Autodesk Inventor part; units mm, degrees
ref_plane "YZ Plane" through (0, 0, 0) normal (1, 0, 0) x (0, 1, 0)
ref_plane "XZ Plane" through (0, 0, 0) normal (0, 1, 0) x (-1, 0, 0)
ref_plane "XY Plane" through (0, 0, 0) normal (0, 0, 1) x (1, 0, 0)
sketch "Sketch1" plane through (0, 0, 0) normal (0, 0, 1) x (1, 0, 0)
  line L0 (-77.055, 89.1324) -> (76.1519, 89.1324)
  line L1 (139.6519, 27.5351) -> (139.6519, -25.4)
  line L2 (76.2, -88.852) -> (-88.4125, -88.852)
  line L3 (-139.7639, 88.9233) -> (139.6519, -88.852) construction
  line L4 (139.6519, 89.1324) -> (-139.2125, -88.852) construction
  line L5 (139.6519, 0.1402) -> (139.6519, 27.5351)
  line L6 (139.6519, 0.1402) -> (139.6519, -25.4)
  line L7 (139.6519, 0.1402) -> (139.6519, -25.4)
  line L8 (139.6519, -25.4) -> (76.2, -88.852)
  line L9 (139.6519, 27.5351) -> (76.1519, 89.1324)
  arc A0 (-139.0653, -41.9162) -> (-88.4125, -88.852) centre (-88.4125, -38.052) ccw
  line L10 (-137.5184, -35.1177) -> (-101.1125, 27.9391)
  line L11 (-139.2125, -38.052) -> (-66.4007, -38.052) construction
  line L12 (-101.1125, 27.9391) -> (-101.1125, 65.0749)
  arc A1 (-137.5184, -35.1177) -> (-139.0653, -41.9162) centre (-127.298, -41.0185) ccw
  line L13 (-77.055, 89.1324) -> (-101.1125, 65.0749)
  line L14 (-77.055, 89.1324) -> (-42.3901, 89.1324) construction
  point P0 (0, 0)
  dimension "d9" = 50.8
extrude "Extrusion1" add sketch "Sketch1" along normal mid plane 203.2
sketch "Sketch2" plane through (-77.055, 89.1324, 101.6) normal (0, 1, 0) x (1, 0, 0)
  circle A0 centre (77.055, 101.6) radius 25.4
  dimension "d16" = 50.8
extrude "Extrusion2" cut sketch "Sketch2" against normal blind 38.1
sketch "Sketch4" plane through (0, 0, 101.6) normal (0, 0, 1) x (1, 0, 0)
  circle A0 centre (0, 0) radius 19.05
  dimension "d22" = 38.1
sketch "Sketch5" plane through (0, 0, -101.6) normal (0, 0, -1) x (-1, 0, 0)
  circle A0 centre (0, 0) radius 19.05
  dimension "d23" = 38.1
extrude "Extrusion4" add sketch "Sketch5" along normal blind 203.2
extrude "Extrusion5" add sketch "Sketch4" along normal blind 203.2
sketch "Sketch6" plane through (-101.1125, 27.9391, 101.6) normal (-1, 0, 0) x (0, 0, 1)
  line L0 (-127, 12.4705) -> (-75.6804, 12.4705)
  line L1 (-127, 12.4705) -> (-76.2, 12.4705)
  line L2 (-76.2, 12.4705) -> (-76.2, -116.9301)
  line L3 (-76.2, -116.9301) -> (-127, -116.9301)
  line L4 (-127, -116.9301) -> (-127, 12.4705)
  point P0 (-101.6, -27.9391)
extrude "Extrusion6" cut sketch "Sketch6" along normal blind 38.1 and the other way blind 19.05
sketch "Sketch7" plane through (-101.1125, 27.9391, -25.4) normal (0, 0, 1) x (1, 0, 0)
  circle A0 centre (-3.8712, -78.6483) radius 12.7
  point P0 (101.1125, -27.9391)
  dimension "d34" = 25.4
extrude "Extrusion7" add sketch "Sketch7" along normal blind 50.8
sketch "Sketch8" plane through (-101.1125, 27.9391, -25.4) normal (0, 0, 1) x (1, 0, 0)
  line L0 (19.05, -116.7911) -> (19.05, 12.4705)
  arc A0 (19.05, -116.7911) -> (19.05, 12.4705) centre (-100.0567, -52.1603) ccw
  point P0 (101.1125, -27.9391)
extrude "Extrusion8" cut sketch "Sketch8" along normal blind 50.8
sketch "Sketch10" plane through (0, 51.0324, 0) normal (0, 1, 0) x (1, 0, 0)
  circle A0 centre (0, 0) radius 25.4
  circle A1 centre (0, 0) radius 31.75
  dimension "d42" = 63.5
extrude "Extrusion10" cut sketch "Sketch10" along normal blind 5.08
properties part number "center piece"
Geometry check sheet. Reference: the model listing, model coordinates, mm. A direction names the side the tool comes from. Give positions to 0.01 mm unless a question says otherwise; leave off trailing zeros. Order: outer loops, then holes, each group sorted by start corner. A loop starts at its lowest first (then second) coordinate and runs counter-clockwise, first axis right, second up.
1. Sectioned sample at B-B (y = 0). Record the boundary of the cut face in (x, z), then the cut area to 3 significant figures.
Completed:
outline: (-117.24, -101.6) - (-19.05, -101.6) - (-19.05, -304.8) - (19.05, -304.8) - (19.05, -101.6) - (139.65, -101.6) - (139.65, 101.6) - (19.05, 101.6) - (19.05, 304.8) - (-19.05, 304.8) - (-19.05, 101.6) - (-117.24, 101.6) - (-117.24, 25.4) - (-67.84, 25.4) - (-67.84, -25.4) - (-117.24, -25.4) - close
area: 65,200 mm2
2. Draft check along X on faces 3 (the face through (-88.92, 77.27, -1.42)), 4 (the face through (0, 51.032, 0)), 5 (the face through (-6.883, 53.537, -30.995)), 6 (the face through (108.37, -56.68, -1.42)). Enter one of: pulls with the +X half, pulls with the -X half, needs draft (parallel to the pull), parting line crosses it, or undercut.
Completed:
face 3: pulls with the -X half
face 4: undercut
face 5: undercut
face 6: pulls with the +X half
3. Sectioned sample at A-A (x = 0). Record the boundary of the cut face in (y, z), then the cut area to 3 significant figures.
Completed:
outline: (-88.85, -101.6) - (-19.05, -101.6) - (-19.05, -304.8) - (19.05, -304.8) - (19.05, -101.6) - (89.13, -101.6) - (89.13, -25.4) - (56.11, -25.4) - (56.11, -31.75) - (51.03, -31.75) - (51.03, 31.75) - (56.11, 31.75) - (56.11, 25.4) - (89.13, 25.4) - (89.13, 101.6) - (19.05, 101.6) - (19.05, 304.8) - (-19.05, 304.8) - (-19.05, 101.6) - (-88.85, 101.6) - close
area: 49,700 mm2
4. Sectioned sample at D-D (x = -55). Record the boundary of the cut face in (y, z), then the cut area to 3 significant figures.
Completed:
outline: (-88.85, -101.6) - (89.13, -101.6) - (89.13, 101.6) - (-88.85, 101.6) - close
area: 36,200 mm2
5. Scan lines: line 1 (Z direction, x = 0, y = 67.5); line 2 (Z direction, x = 0, y = 52.9); line 3 (Z direction, x = -23, y = -45). Record each from-to range of solid material in increasing order.
Completed:
line 1: z = -101.6 to -25.4, 25.4 to 101.6
line 2: z = -101.6 to -31.75, 31.75 to 101.6
line 3: z = -101.6 to 101.6
6. Depth check by flat-ended pin: pin 1 (6 mm diameter, centred on x = -65.5, y = 36, fed in from -Z); pin 2 (10 mm diameter, centred on x = -74.5, y = -61.5, fed in from +Z); pin 3 (1.5 mm diameter, centred on y = 15.5, z = 206.5, fed in from -X). Enter the tip coordinate at first touch or a pass-through.
Completed:
pin 1: stops at z = -101.6
pin 2: stops at z = 101.6
pin 3: stops at x = -12.06
7. Access from +Z, -Z, +X, -X, +Y, -Y to the whole of each face (thin tool, end or side, straight path). Record for faces 1 (the face through (-65.66, -23.28, -0.36)), 2 (the face through (-122.55, -75.67, 62.97)).
Completed:
face 1: none
face 2: +Z, -Z, -X, -Y
8. Sectioned sample at C-C (z = 233.5). Record the boundary of the cut face in (x, y), then the cut area to 3 significant figures.
Completed:
outline: circle Ø38.1 at (0, 0)
area: 1,140 mm2
